The model under review builds one solid part; all positions refer to its coordinate system, in mm. Face numbers are marked on the shaded views. A direction names the side the tool comes from. Give positions to 0.01 mm unless a question says otherwise; leave off trailing zeros. Order: outer loops, then holes, each group sorted by start corner. A loop starts at its lowest first (then second) coordinate and runs counter-clockwise, first axis right, second up. Notation, with made-up numbers: M 31.5,0.25 L 85.5,0.25 A20 ccw 85.5,5.25 Z; hole C 22,-14.75 d7. An arc over 180 degrees is marked long. One line per question, with ' | ' between items. Start each with the question number.
1. For the marked faces 1 and 2, list the 3-axis set-ups (+Z, -Z, +X, -X, +Y, -Y) from which the entire face can be reached by the end or side of a thin tool; tool diameter is ignored.
2. We need section C-C on z = 14. Write out the cut boundary in (x, y), then the cut area to 3 significant figures.
3. Insertion check: P1, Ø12, axis at x = -25, y = 39, coming from the +Z side; P2, Ø6, axis at x = -32, y = -3, coming from the +Z side; P3, Ø12, axis at x = -34, z = 16.5, coming from the -Y side. Each pin has a flat end and moves straight along its axis. Give the tip position at first contact, or say it passes through.
4. The part is to be moulded in two halves that separate along Z. For the marked faces 3, 4 and 5, say which applies: +Z half, -Z half, draft (parallel to the pull), parting line (faces both ways), or undercut.
5. Wall thickness on L1, parallel to Z at x = -4.5, y = 47; L2, parallel to X at y = 3.5, z = 22.5; L3, parallel to Y at x = -25.5, z = 27.5: over which ranges is each line inside the solid? List them lowest first.
6. We need section B-B on y = 30. Write out the cut boundary in (x, z).
7. We need section D-D on y = 42. Write out the cut boundary in (x, z).
8. We need section A-A on x = -33. Write out the cut boundary in (y, z) (3 decimals).
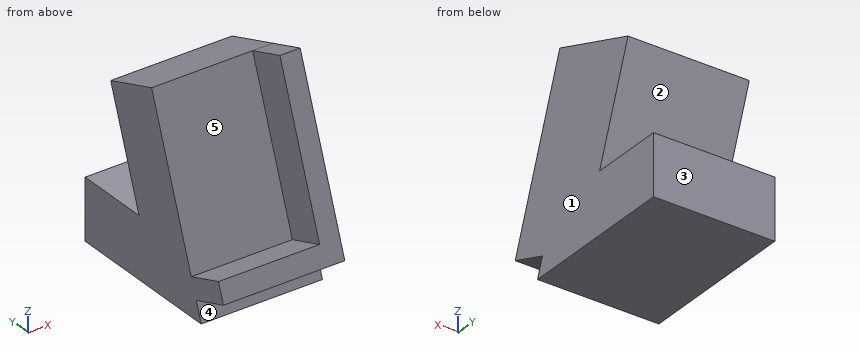
```python
from build123d import *

# Parameters (mm, degrees)
F1_DEPTH = 38.1
F3_DEPTH = 12.7


with BuildPart() as f1:
    # F0 (on Right) → F1 (new body)
    with BuildSketch(Plane.YZ):
        Polygon((21.7182791012, 59.6704814199), (0, 0), (50.8, 0), (50.8, 19.05), (27.2062195284, 19.05), (39.6194235272, 53.1549976896), align=None)
    extrude(amount=-F1_DEPTH)

    # F2 (on face) → F3 (join)
    with BuildSketch(Plane(origin=(0, 0, 0), x_dir=(1, 0, 0), z_dir=(0, -0.9396926208, 0.3420201433))):
        Polygon((0, 6.35), (0, 63.5), (-6.35, 63.5), (-6.35, 12.7), (-38.1, 12.7), (-38.1, 6.35), align=None)
    extrude(amount=F3_DEPTH)


solid = f1.part
```
Entries:
1) face 1: +Z, -Z, +X, +Y, -Y | face 2: +X, -X, +Y
2) outline: M -38.1,-8.42 L 0,-8.42 L 0,50.8 L -38.1,50.8 L -38.1,5.1 L -6.35,5.1 L -6.35,-1.33 L -38.1,-1.33 Z | area: 2,050 mm^2
3) P1: stops at z = 55.56 | P2: stops at z = 15.7 | P3: stops at y = -9.69
4) face 3: draft | face 4: undercut | face 5: +Z half
5) L1: z = 0 to 19.05 | L2: x = -6.35 to 0 | L3: y = 10.01 to 30.28
6) outline: M -38.1,0 L 0,0 L 0,19.05 L -38.1,19.05 Z; M -38.1,26.73 L 0,26.73 L 0,56.66 L -38.1,56.66 Z
7) outline: M -38.1,0 L 0,0 L 0,19.05 L -38.1,19.05 Z
8) outline: M -9.762,10.311 L 2.172,5.967 L 0,0 L 50.8,0 L 50.8,19.05 L 27.206,19.05 L 39.619,53.155 L 21.718,59.67 L 4.344,11.934 L -7.59,16.278 Z
